Geometry check sheet. Reference: drawing and pictorial views, mm from the part's lowest x, y, z. A direction names the side the tool comes from. Give positions to 0.01 mm unless a question says otherwise; leave off trailing zeros. Write each loop counter-clockwise with the first axis right and the second up, starting at its lowest first coordinate (ties: lowest second). Pieces come first, ordered by that corner, then holes. Notation, with made-up numbers: (16, -9.5) - (42, -9.5) arc R25 ccw to (42, 19.5) - close; hole circle Ø8 at (-36.5, -36.5). An arc over 180 degrees is marked (long way). Write item = value, one per line. Start each with the question number.
(1) Section check D-D, the plane y = 12.75. Enter the section's corners in (x, z), plus the area to 3 significant figures.
(2) Section check C-C, the plane x = 28. Enter the section's corners in (y, z).
(3) Section check B-B, the plane z = 3. Enter the section's corners in (x, y), plus the area to 3 significant figures.
(4) Depth check by flat-ended pin: pin 1 Ø1 at (x, z) = (19.5, 5) entering from +Y; pin 2 Ø3 at (x, y) = (9, 8.5) entering from -Z. Enter the tip coordinate at first touch or a pass-through.
(5) Section check A-A, the plane y = 4. Enter the section's corners in (x, z), plus the area to 3 significant figures.
(6) Access from +Z, -Z, +X, -X, +Y, -Y to the whole of each face (thin tool, end or side, straight path). Record for the marked faces 1 and 2.
(7) Thickness scan on L1, parallel to Y at x = 8, z = 7.55; L2, parallel to Y at x = 35.3, z = 3; L3, parallel to X at y = 12, z = 2.75. Record the ranges inside material, lowest first.
(8) Draft check along X on the marked faces 3, 4 and 5. Enter one of: pulls with the +X half, pulls with the -X half, needs draft (parallel to the pull), parting line crosses it, or undercut.
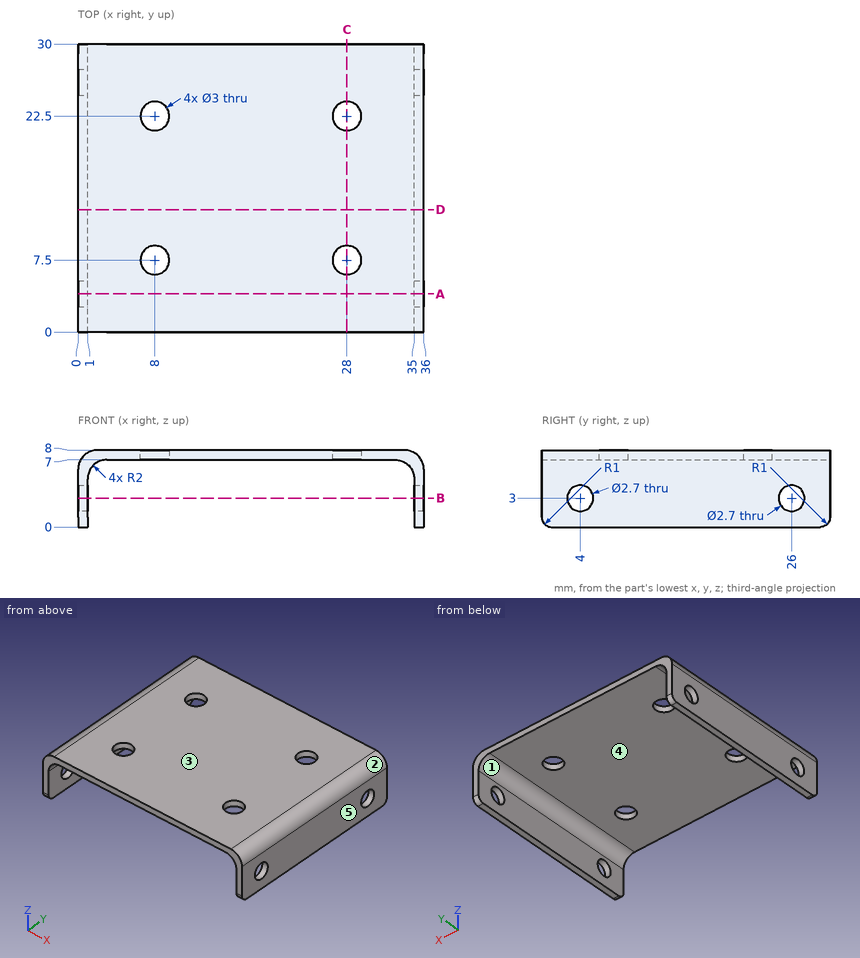
Model answer:
q1.outline = (0, 0) - (1, 0) - (1, 5) arc R2 cw to (3, 7) - (33, 7) arc R2 cw to (35, 5) - (35, 0) - (36, 0) - (36, 6) arc R2 ccw to (34, 8) - (2, 8) arc R2 ccw to (0, 6) - close
q1.area = 50.0 mm²
q2.outline = (0, 7) - (6, 7) - (6, 8) - (0, 8) - close; (9, 7) - (21, 7) - (21, 8) - (9, 8) - close; (24, 7) - (30, 7) - (30, 8) - (24, 8) - close
q3.outline = (0, 0) - (1, 0) - (1, 2.65) - (0, 2.65) - close; (0, 5.35) - (1, 5.35) - (1, 24.65) - (0, 24.65) - close; (0, 27.35) - (1, 27.35) - (1, 30) - (0, 30) - close; (35, 0) - (36, 0) - (36, 2.65) - (35, 2.65) - close; (35, 5.35) - (36, 5.35) - (36, 24.65) - (35, 24.65) - close; (35, 27.35) - (36, 27.35) - (36, 30) - (35, 30) - close
q3.area = 49.2 mm²
q4.pin_1 = through
q4.pin_2 = 7
q5.outline = (0, 0) - (1, 0) - (1, 1.65) - (0, 1.65) - close; (0, 4.35) - (1, 4.35) - (1, 5) arc R2 cw to (3, 7) - (33, 7) arc R2 cw to (35, 5) - (35, 4.35) - (36, 4.35) - (36, 6) arc R2 ccw to (34, 8) - (2, 8) arc R2 ccw to (0, 6) - close; (35, 0) - (36, 0) - (36, 1.65) - (35, 1.65) - close
q5.area = 44.6 mm²
q6.face_1 = -Z, +Y, -Y
q6.face_2 = +Z, +X, +Y, -Y
q7.L1 = 0 to 6, 9 to 21, 24 to 30
q7.L2 = 0 to 2.65, 5.35 to 24.65, 27.35 to 30
q7.L3 = 0 to 1, 35 to 36
q8.face_3 = needs draft
q8.face_4 = undercut
q8.face_5 = pulls with the +X half
